Work out the finished part from the listing and answer in its coordinate system (mm). A direction names the side the tool comes from. Give positions to 0.01 mm unless a question says otherwise; leave off trailing zeros. Loops run counter-clockwise (first coordinate to the right, second up) from the corner with the lowest first, then second, coordinate; pieces in that order, holes last. Notation, with made-up numbers: (65, 37) -> (79, 37) arc R22 cw to (79, 73) -> close; hole circle Ø10 at (-25, 42.5). An arc over 180 degrees is marked (long way). Answer as CSV lines item,"result". Start each with the question number.
1. Find section B-B, the plane z = -5. Give the vertices of the cut face in (x, y), and give its area (3 significant figures).
2. Find section A-A, the plane x = 19.05. Give the vertices of the cut face in (y, z), and give its area (3 significant figures).
3. Find section D-D, the plane z = 1. Give the vertices of the cut face in (x, y), and give its area (3 significant figures).
4. A tool of negligible diameter and unlimited length cuts with its end or side. For faces 1 (the face through (-19.045, -0.419, 15.927)), 2 (the face through (16, -6.35, 15)), from which of +Z, -Z, +X, -X, +Y, -Y can it reach the whole face along a straight path? Write none if from no direction.
5. Find section C-C, the plane x = 5. Give the vertices of the cut face in (y, z), and give its area (3 significant figures).
6. Find the intervals of material crossed by line 1 along Z through (x, y) = (19, -10); line 2 along Y through (x, z) = (7.5, 21); line 3 along Y through (x, z) = (-4, 34), in increasing order.
7. Flat-ended cylindrical pins translate along their axes: pin 1 Ø8 at (y, z) = (11, 20.5) entering from -X; pin 2 Ø10 at (y, z) = (-4.5, -1) entering from +X; pin 3 Ø15 at (x, z) = (46, 8.5) entering from -Y. Find the tip coordinate at first contact, or state that the pin passes through.
8. Determine the mould class of faces 3 (the face through (12, 8, -9.828)), 4 (the face through (31.75, -13, 16)), 5 (the face through (17.588, 12.611, 21.686)) for opening direction Z: +Z half, -Z half, draft (parallel to the pull), parting line (faces both ways), or undercut.
from build123d import *

# Parameters (mm, degrees)
F0_W          = 12.7
F0_H          = 50.8
F1_ANGLE_BACK = 90
F1_ANGLE      = 180
F2_DEPTH      = 63.5
F3_DEPTH      = 31.75
F5_D          = 13.49248


with BuildPart() as f1:
    # F0 (on Front) → F1 (revolve)
    with BuildSketch(Plane.XZ, mode=Mode.PRIVATE) as f1_sk:
        with Locations((-12.7, 15.5715065134)):
            Rectangle(F0_W, F0_H)
    revolve(f1_sk.sketch.rotate(Axis((0, 0, 15.5715065134), (0, 0, -1)), -F1_ANGLE_BACK), axis=Axis((0, 0, 15.5715065134), (0, 0, -1)), revolution_arc=F1_ANGLE)

    # F2 (add): a face of the model
    f2_faces = [f1.faces().sort_by_distance(p)[0] for p in [
        (0, 12.7, 15.5715065134),
    ]]
    extrude(f2_faces, amount=F2_DEPTH)

    # F3 (add): a face of the model
    f3_faces = [f1.faces().sort_by_distance(p)[0] for p in [
        (0, -12.7, 15.5715065134),
    ]]
    extrude(f3_faces, amount=F3_DEPTH)

    # F5 (through all)
    with Locations(Plane(origin=(0, 19.05, 0), x_dir=(-1, 0, 0), z_dir=(0, 1, 0))):
        with Locations((-19.05, 2.8715065134), (-19.05, 28.2715065134)):
            Hole(F5_D / 2)


solid = f1.part
Resolved:
1,outline,"(0, -19.05) -> (31.75, -19.05) -> (31.75, -6.35) -> (0, -6.35) arc R6.35 cw to (0, 6.35) -> (63.5, 6.35) -> (63.5, 19.05) -> (0, 19.05) arc R19.05 ccw to start"
1,area,"1,720 mm^2"
2,outline,"(-19.05, -9.83) -> (-6.35, -9.83) -> (-6.35, -3.87) -> (-19.05, -3.87) -> close; (-19.05, 9.62) -> (-6.35, 9.62) -> (-6.35, 21.53) -> (-19.05, 21.53) -> close; (-19.05, 35.02) -> (-6.35, 35.02) -> (-6.35, 40.97) -> (-19.05, 40.97) -> close; (6.35, -9.83) -> (19.05, -9.83) -> (19.05, -3.87) -> (6.35, -3.87) -> close; (6.35, 9.62) -> (19.05, 9.62) -> (19.05, 21.53) -> (6.35, 21.53) -> close; (6.35, 35.02) -> (19.05, 35.02) -> (19.05, 40.97) -> (6.35, 40.97) -> close"
2,area,"605 mm^2"
3,outline,"(0, -19.05) -> (12.57, -19.05) -> (12.57, -6.35) -> (0, -6.35) arc R6.35 cw to (0, 6.35) -> (12.57, 6.35) -> (12.57, 19.05) -> (0, 19.05) arc R19.05 ccw to start; (25.53, -19.05) -> (31.75, -19.05) -> (31.75, -6.35) -> (25.53, -6.35) -> close; (25.53, 6.35) -> (63.5, 6.35) -> (63.5, 19.05) -> (25.53, 19.05) -> close"
3,area,"1,390 mm^2"
4,face 1,"+Z, -Z, -X"
4,face 2,"+Z, -Z, +X"
5,outline,"(-19.05, -9.83) -> (-6.35, -9.83) -> (-6.35, 40.97) -> (-19.05, 40.97) -> close; (6.35, -9.83) -> (19.05, -9.83) -> (19.05, 40.97) -> (6.35, 40.97) -> close"
5,area,"1,290 mm^2"
6,line 1,"z = -9.83 to -3.87, 9.62 to 21.53, 35.02 to 40.97"
6,line 2,"y = -19.05 to -6.35, 6.35 to 19.05"
6,line 3,"y = -18.63 to -4.93, 4.93 to 18.63"
7,pin 1,"stops at x = -17.72"
7,pin 2,"stops at x = 31.75"
7,pin 3,"stops at y = 6.35"
8,face 3,"-Z half"
8,face 4,"draft"
8,face 5,"undercut"
